For this review, take the finished solid that the model builds, in its own axes (mm). Face numbers are marked on the shaded views. A direction names the side the tool comes from. Coordinates: 2 decimals unless noted, no trailing zeros. Loops run counter-clockwise (first coordinate to the right, second up) from the corner with the lowest first, then second, coordinate; pieces in that order, holes last. Notation, with made-up numbers: M 14,-14.75 L 46,-14.75 A28 cw 46,11.25 Z; hole C 20.25,5 d7. An arc over 180 degrees is marked long. Write each question's results on one line, items separated by ' | '. Start each with the question number.
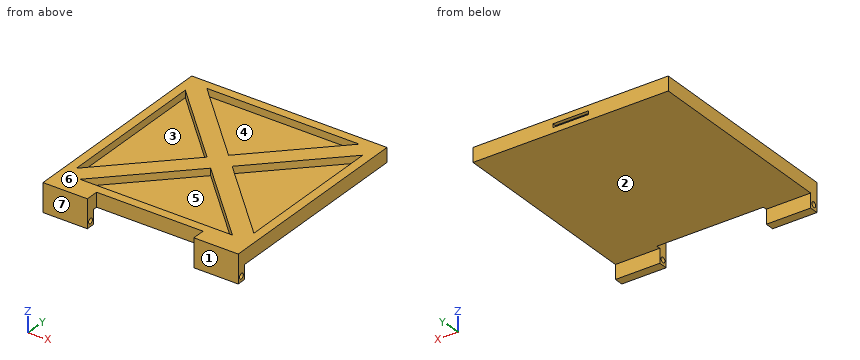
```python
from build123d import *

# Parameters (mm, degrees)
SKETCH2_W               = 110
SKETCH2_H               = 110
BOSS_EXTRUDE1_DEPTH     = 8
BOSS_EXTRUDE2_DEPTH     = 25
CUT_EXTRUDE1_DEPTH      = 127.645420367
CUT_EXTRUDE1_DEPTH_BACK = 127.645420367
SKETCH10_R              = 1.5
CUT_EXTRUDE2_DEPTH      = 4
SKETCH12_W              = 20
SKETCH12_H              = 2
CUT_EXTRUDE3_DEPTH      = 2


with BuildPart() as part:
    # Sketch2 → Boss-Extrude1 (new body)
    with BuildSketch(Plane.XY):
        Rectangle(SKETCH2_W, SKETCH2_H)
    extrude(amount=BOSS_EXTRUDE1_DEPTH)

    # Sketch8 → Boss-Extrude2 (add)
    with BuildSketch(Plane(origin=(55, 0, 0), x_dir=(0, 0, -1), z_dir=(1, 0, 0))):
        Polygon((-8, -55), (-8, -62.25), (8, -62.25), (8, -57.25), (0, -57.25), (0, -55), align=None)
    boss_extrude2 = extrude(amount=-BOSS_EXTRUDE2_DEPTH)

    # Mirror1: Boss-Extrude2 across plane
    add(boss_extrude2.mirror(Plane(origin=(0, 0, 0), x_dir=(0, 0, 1), z_dir=(1, 0, 0))))

    # Sketch10 → Cut-Extrude1 (cut, two sides: drawn at the far end of the back side and taken through both)
    with BuildSketch(Plane.ZY.offset(55).offset(-CUT_EXTRUDE1_DEPTH_BACK)):
        with Locations((-5, -59.762907668)):
            Circle(SKETCH10_R)
    extrude(amount=CUT_EXTRUDE1_DEPTH + CUT_EXTRUDE1_DEPTH_BACK, mode=Mode.SUBTRACT)

    # Sketch11 → Cut-Extrude2 (cut)
    with BuildSketch(Plane.XY.offset(8)):
        Polygon((-42.928932188, 50), (0, 7.071067812), (42.928932188, 50), align=None)
        Polygon((50, -42.928932188), (50, 42.928932188), (7.071067812, 0), align=None)
        Polygon((-42.928932188, -50), (42.928932188, -50), (0, -7.071067812), align=None)
        Polygon((-50, 42.928932188), (-50, -42.928932188), (-7.071067812, 0), align=None)
    extrude(amount=-CUT_EXTRUDE2_DEPTH, mode=Mode.SUBTRACT)

    # Sketch12 → Cut-Extrude3 (cut)
    with BuildSketch(Plane(origin=(0, 55, 0), x_dir=(1, 0, 0), z_dir=(0, 1, 0))):
        with Locations((0, -4)):
            Rectangle(SKETCH12_W, SKETCH12_H)
    extrude(amount=-CUT_EXTRUDE3_DEPTH, mode=Mode.SUBTRACT)


solid = part.part
```
Q1. Take a section at D-D, the plane x = -39. Give the boundary of the cut face in (y, z), then the cut area to 3 significant figures.
Q2. To check wall thickness, follow line 1 along Y through (x, z) = (36, -5.25); line 2 along Y through (x, z) = (48.25, -5); line 3 along Y through (x, z) = (-27, 4.25). State the ranges of each line that lie inside material, in increasing order.
Q3. Take a section at C-C, the plane x = 14.5. Give the boundary of the cut face in (y, z).
Q4. For the marked faces 1, 2 and 3, list the 3-axis set-ups (+Z, -Z, +X, -X, +Y, -Y) from which the entire face can be reached by the end or side of a thin tool; tool diameter is ignored.
Q5. The part is to be moulded in two halves that separate along Y. For the marked faces 4, 5, 6 and 7, say which applies: pulls with the +Y half, pulls with the -Y half, needs draft (parallel to the pull), parting line crosses it, or undercut.
Q6. Take a section at B-B, the plane y = 5. Give the boundary of the cut face in (x, z).
Q7. Insertion check: P1, Ø3, axis at x = 11.5, y = -15, coming from the -Z side; P2, Ø13, axis at x = -7.5, y = -25, coming from the +Z side; P3, Ø2.5, axis at y = -59.76, z = -5, coming from the +X side; P4, Ø6, axis at x = 18, z = 2.5, coming from the -Y side. Each pin has a flat end and moves straight along its axis. Give the tip position at first contact, or say it passes through.
Q8. Take a section at A-A, the plane z = -1.5. Give the boundary of the cut face in (x, y).
Results:
1) outline: M -62.25,-8 L -57.25,-8 L -57.25,0 L 55,0 L 55,8 L 50,8 L 50,4 L 46.07,4 L 46.07,8 L 31.93,8 L 31.93,4 L -31.93,4 L -31.93,8 L -46.07,8 L -46.07,4 L -50,4 L -50,8 L -62.25,8 Z; hole C -59.76,-5 d3 | area: 684 mm^2
2) line 1: -62.25 to -61.24, -58.28 to -57.25 | line 2: -62.25 to -61.26, -58.26 to -57.25 | line 3: -55 to -50, -34.07 to -19.93, 19.93 to 34.07, 50 to 55
3) outline: M -55,0 L 55,0 L 55,8 L 50,8 L 50,4 L 21.57,4 L 21.57,8 L 7.43,8 L 7.43,4 L -7.43,4 L -7.43,8 L -21.57,8 L -21.57,4 L -50,4 L -50,8 L -55,8 Z
4) face 1: +Z, -Z, +X, -X, -Y | face 2: -Z, +X, -X, +Y | face 3: +Z
5) face 4: undercut | face 5: undercut | face 6: needs draft | face 7: pulls with the -Y half
6) outline: M -55,0 L 55,0 L 55,8 L 50,8 L 50,4 L 12.07,4 L 12.07,8 L -12.07,8 L -12.07,4 L -50,4 L -50,8 L -55,8 Z
7) P1: z = 0 | P2: z = 4 | P3: through | P4: y = -55
8) outline: M -55,-62.25 L -30,-62.25 L -30,-57.25 L -55,-57.25 Z; M 30,-62.25 L 55,-62.25 L 55,-57.25 L 30,-57.25 Z
